Autodesk Inventor part; units mm, degrees
ref_plane "YZ Plane" through (0, 0, 0) normal (1, 0, 0) x (0, 1, 0)
ref_plane "XZ Plane" through (0, 0, 0) normal (0, 1, 0) x (-1, 0, 0)
ref_plane "XY Plane" through (0, 0, 0) normal (0, 0, 1) x (1, 0, 0)
sketch "Sketch1" plane through (0, 0, 0) normal (0, 0, 1) x (1, 0, 0)
  arc A0 (-1.25, 1) -> (-3.25, 0) centre (-2, 0) ccw
  line L0 (0, 1) -> (-1.25, 1)
  line L1 (0, 0) -> (-3.25, 0)
  line L2 (0, 1) -> (0, 0) construction
  arc A1 (3.25, 0) -> (1.25, 1) centre (2, 0) ccw
  line L3 (0, 1) -> (1.25, 1)
  line L4 (0, 0) -> (3.25, 0)
  dimension "d0" = 2.5
  dimension "d2" = 1
  dimension "d5" = 0
  dimension "d6" = 0
  dimension "d11" = 3.25
revolve "Revolution1" add sketch "Sketch1" angle 360 about axis through (0, 0, 0) along (1, 0, 0)
sketch "Sketch2" plane through (0, 0, 0) normal (0, 0, 1) x (1, 0, 0)
  line L0 (-3.31, 0) -> (3.31, 0)
  line L1 (3.81, -0.5) -> (3.81, -4.25)
  line L2 (-3.81, -0.5) -> (-3.81, -4.25)
  arc A0 (-3.31, 0) -> (-3.81, -0.5) centre (-3.31, -0.5) ccw
  arc A1 (3.81, -0.5) -> (3.31, 0) centre (3.31, -0.5) ccw
  point P0 (0, 0)
  dimension "d8" = 4.25
  dimension "d9" = 7.62
  dimension "d10" = 3.81
  dimension "d12" = 0.5
  dimension "d13" = 0
  dimension "d14" = 4.25
sketch "Sketch3" plane through (0, 0, 0) normal (1, 0, 0) x (0, 1, 0)
  circle A0 centre (0, 0) radius 0.25
  dimension "d15" = 0.5
sweep "Sweep1" add profiles "Sketch3" path "Sketch2"
equation "\"d14\" = d8"
properties part number "Resistor"
Could you check a few things on this model? Use its own coordinates, in mm. Give positions to 0.01 mm unless a question says otherwise; leave off trailing zeros. Order: outer loops, then holes, each group sorted by start corner. A loop starts at its lowest first (then second) coordinate and runs counter-clockwise, first axis right, second up. Notation, with made-up numbers: (0, -24.5) -> (35, -24.5) arc R13 ccw to (35, -12.5) -> close; hole circle Ø7 at (6, 46.5). An arc over 180 degrees is marked (long way). Return JSON: item names as keys, results as strings.
1. Imagine slicing it at D-D on x = 0. List the corners of the cut face in (y, z) for me.
Answer list:
{"outline": "circle Ø2 at (0, 0)"}
2. Imagine slicing it at B-B on y = -2.9. List the corners of the cut face in (x, z) for me.
Answer list:
{"outline": "circle Ø0.5 at (-3.81, 0); circle Ø0.5 at (3.81, 0)"}
3. I need wall thicknesses on line 1 (Y direction, x = -2.75, z = 0.05); line 2 (X direction, y = 0.95, z = 0.4); line 3 (X direction, y = 0.15, z = -0.6). Which ranges of each line are inside material? Lowest first, please. Write a range as from..to.
Answer list:
{"line 1": "y = -1..1", "line 2": "x = -2.71..-1.29, 1.29..2.71", "line 3": "x = -3.09..3.09"}
4. Imagine slicing it at A-A on z = 0. List the corners of the cut face in (x, y) for me.
Answer list:
{"outline": "(-4.06, -4.25) -> (-3.56, -4.25) -> (-3.56, -0.5) arc R0.25 cw to (-3.31, -0.25) -> (-3.22, -0.25) arc R1.25 ccw to (-1.25, -1) -> (1.25, -1) arc R1.25 ccw to (3.22, -0.25) -> (3.31, -0.25) arc R0.25 cw to (3.56, -0.5) -> (3.56, -4.25) -> (4.06, -4.25) -> (4.06, -0.5) arc R0.75 ccw to (3.31, 0.25) -> (3.22, 0.25) arc R1.25 ccw to (1.25, 1) -> (-1.25, 1) arc R1.25 ccw to (-3.22, 0.25) -> (-3.31, 0.25) arc R0.75 ccw to (-4.06, -0.5) -> close"}
5. Imagine slicing it at C-C on y = -0.9. List the corners of the cut face in (x, z) for me, then the cut area to 3 significant figures.
Answer list:
{"outline": "circle Ø0.5 at (-3.81, 0); (-1.25, -0.44) -> (1.25, -0.44) arc R0.87 ccw (long way) to (1.25, 0.44) -> (-1.25, 0.44) arc R0.87 ccw (long way) to start; circle Ø0.5 at (3.81, 0)", "area": "7.16 mm2"}
